Autodesk Inventor part; units mm, degrees
ref_plane "YZ Plane" through (0, 0, 0) normal (1, 0, 0) x (0, 1, 0)
ref_plane "XZ Plane" through (0, 0, 0) normal (0, 1, 0) x (-1, 0, 0)
ref_plane "XY Plane" through (0, 0, 0) normal (0, 0, 1) x (1, 0, 0)
sketch "Sketch1" plane through (0, 0, 0) normal (0, 1, 0) x (-1, 0, 0)
  line L0 (50, 100) -> (-50, 100)
  line L1 (-50, 100) -> (-50, -100)
  line L2 (-50, -100) -> (50, -100)
  line L3 (50, -100) -> (50, 100)
  line L4 (50, 100) -> (-50, -100) construction
  line L5 (-50, 100) -> (50, -100) construction
  point P0 (0, 0)
  dimension "d0" = 100
  dimension "d1" = 200
extrude "Extrusion1" add sketch "Sketch1" along normal blind 5
sketch "Sketch2" plane through (0, 5, 0) normal (0, 1, 0) x (1, 0, 0)
  line L0 (-34.6, -58) -> (34.6, -58)
  line L1 (34.6, -58) -> (34.6, 58)
  line L2 (34.6, 58) -> (-34.6, 58)
  line L3 (-34.6, 58) -> (-34.6, -58)
  line L4 (-34.6, -58) -> (34.6, 58) construction
  line L5 (34.6, -58) -> (-34.6, 58) construction
  circle A0 centre (-12.9, 54.5) radius 2.5
  circle A1 centre (15.1, 54.5) radius 2.5
  line L6 (0, 0) -> (-70, 0) construction
  line L7 (0, 0) -> (70, 0) construction
  circle A2 centre (-12.9, -54.5) radius 2.5
  circle A3 centre (15.1, -54.5) radius 2.5
  dimension "d4" = 69.2
  dimension "d5" = 116
  dimension "d6" = 19.5
  dimension "d7" = 28
  dimension "d8" = 3.5
  dimension "d9" = 3.5
  dimension "d10" = 5
  dimension "d11" = 5
  dimension "d12" = 70
  dimension "d13" = 180
hole "Hole1" at (-12.9, 5, 54.5) at (15.1, 5, 54.5) at (-12.9, 5, -54.5) at (15.1, 5, -54.5) direction (0, -1, 0) diameter 4.4587 end through all
sketch "Sketch3" plane through (0, 5, 0) normal (0, 1, 0) x (1, 0, 0)
  line L0 (-34.6, -81) -> (34.6, -81)
  line L1 (34.6, -81) -> (34.6, 81)
  line L2 (34.6, 81) -> (-34.6, 81)
  line L3 (-34.6, 81) -> (-34.6, -81)
  line L4 (-34.6, -81) -> (34.6, 81) construction
  line L5 (34.6, -81) -> (-34.6, 81) construction
  point P0 (0, 0)
  point P1 (15.1, -73.5)
  point P2 (-12.9, -73.5)
  dimension "d21" = 69.2
  dimension "d22" = 162
  dimension "d23" = 7.5
  dimension "d24" = 7.5
  dimension "d25" = 28
  dimension "d26" = 19.5
hole "Hole2" at (15.1, 5, 73.5) at (-12.9, 5, 73.5) direction (0, -1, 0) diameter 4.134 end through all
mirror "Mirror2" about plane through (0, 0, 0) normal (0, 0, 1) of "Hole2"
properties part number "Aluminum_Heatsink_Base"
Could you check a few things on this model? Use its own coordinates, in mm. Give positions to 0.01 mm unless a question says otherwise; leave off trailing zeros. Order: outer loops, then holes, each group sorted by start corner. A loop starts at its lowest first (then second) coordinate and runs counter-clockwise, first axis right, second up. Notation, with made-up numbers: (65.5, 8.5) - (102.5, 8.5) arc R13 cw to (102.5, 23.5) - close; hole circle Ø7 at (89.25, 82.5). An arc over 180 degrees is marked (long way). Return JSON: item names as keys, results as strings. Group by question number.
Q1. Suppose I cut it at B-B, the plane x = -12.9. Please give me the cut outline in (y, z).
Q2. Suppose I cut it at A-A, the plane z = 73.5. Please give me the cut outline in (x, y), and give its area (3 significant figures).
Q3. Please list where these lines run through material, in increasing order: line 1 along Z through (x, y) = (15.1, 3.75); line 2 along X through (y, z) = (3.3, 73.5); line 3 along X through (y, z) = (3.7, 54.5). Write a range as [from, to].
Q4. Thinking about a two-plate mould opening in X: for faces 1 (the face through (50, 2, 1)), 2 (the face through (-12.809, 2.465, -71.435)), 3 (the face through (-1, 2, 100)), 4 (the face through (-50, 2, -1)), which applies, pulls with the +X half, pulls with the -X half, needs draft (parallel to the pull), parting line crosses it, or undercut?
Resolved:
{
 "1": {"outline": "(0, -100) - (5, -100) - (5, -75.57) - (0, -75.57) - close; (0, -71.43) - (5, -71.43) - (5, -56.73) - (0, -56.73) - close; (0, -52.27) - (5, -52.27) - (5, 52.27) - (0, 52.27) - close; (0, 56.73) - (5, 56.73) - (5, 71.43) - (0, 71.43) - close; (0, 75.57) - (5, 75.57) - (5, 100) - (0, 100) - close"},
 "2": {"outline": "(-50, 0) - (-14.97, 0) - (-14.97, 5) - (-50, 5) - close; (-10.83, 0) - (13.03, 0) - (13.03, 5) - (-10.83, 5) - close; (17.17, 0) - (50, 0) - (50, 5) - (17.17, 5) - close", "area": "459 mm2"},
 "3": {"line 1": "z = [-100, -75.57], [-71.43, -56.73], [-52.27, 52.27], [56.73, 71.43], [75.57, 100]", "line 2": "x = [-50, -14.97], [-10.83, 13.03], [17.17, 50]", "line 3": "x = [-50, -15.13], [-10.67, 12.87], [17.33, 50]"},
 "4": {"face 1": "pulls with the +X half", "face 2": "undercut", "face 3": "needs draft", "face 4": "pulls with the -X half"}
}
